Input: dimensioned drawing with shaded views. Units: mm. Origin: part minimum x, y, z. A direction names the side the tool comes from. Give positions to 0.01 mm unless a question says otherwise; leave off trailing zeros. Loops run counter-clockwise (first coordinate to the right, second up) from the corner with the lowest first, then second, coordinate; pieces in that order, holes last. Notation, with made-up numbers: M 31,34.5 L 88,34.5 A18 cw 88,44.5 Z; hole C -13.75,59 d9. An arc over 180 degrees is marked long. Answer in a Markdown table with one row per item.
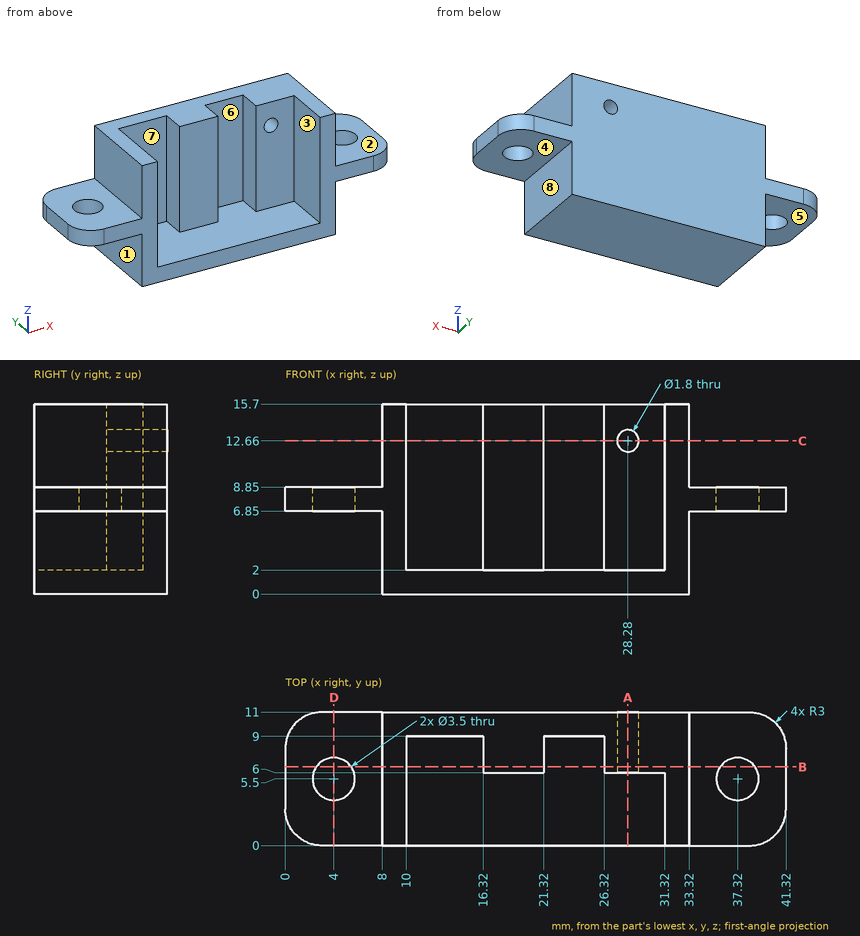
Q1. Section query B-B (y = 6.5). Give the number of separate pieces and of enclosed holes in the cut face, plus the area to 3 significant figures.
Values follow:
| item | result |
|---|---|
| separate pieces | 3 |
| enclosed holes | 1 |
| area | 260 mm^2 |
Q2. Ray query, probe 1 along X at (y, z) = (7.25, 9.25); probe 2 along Z at (x, y) = (28.28, 8.65); probe 3 along X at (y, z) = (3.5, 10.75). Return the intervals inside material, ascending. Write a range as from..to.
Values follow:
| item | result |
|---|---|
| probe 1 | 8..10, 16.32..21.32, 26.32..33.32 |
| probe 2 | 0..11.76, 13.56..15.7 |
| probe 3 | 8..10, 31.32..33.32 |
Q3. Contact query for flat-ended pins moving along their axis: pin 1 Ø4 at (x, z) = (28, 9.5) entering from -Y; pin 2 Ø5.5 at (y, z) = (6, 2.5) entering from -X; pin 3 Ø1.5 at (y, z) = (4, 12) entering from +X. Output: stop coordinate, or through.
Values follow:
| item | result |
|---|---|
| pin 1 | y = 6 |
| pin 2 | x = 8 |
| pin 3 | x = 33.32 |
Q4. Mould query, pull axis X, two halves, no side actions, for the marked faces 5, 6, 7 and 8. Classes: +X half, -X half, draft (parallel to the pull), parting line (faces both ways), or undercut.
Values follow:
| item | result |
|---|---|
| face 5 | draft |
| face 6 | undercut |
| face 7 | undercut |
| face 8 | +X half |
Q5. Section query C-C (z = 12.66). Output: boundary loops of the cut face in (x, y).
Values follow:
| item | result |
|---|---|
| outline | M 8,0 L 10,0 L 10,9 L 16.32,9 L 16.32,6 L 21.32,6 L 21.32,9 L 26.32,9 L 26.32,6 L 27.38,6 L 27.38,11 L 8,11 Z; M 29.18,6 L 31.32,6 L 31.32,0 L 33.32,0 L 33.32,11 L 29.18,11 Z |
Q6. Section query D-D (x = 4). Output: boundary loops of the cut face in (y, z).
Values follow:
| item | result |
|---|---|
| outline | M 0,6.85 L 3.75,6.85 L 3.75,8.85 L 0,8.85 Z; M 7.25,6.85 L 11,6.85 L 11,8.85 L 7.25,8.85 Z |
Q7. Reachability of the marked faces 1, 2, 3 and 4 from +Z, -Z, +X, -X, +Y, -Y: full face, straight path, thin tool, end or side. Return the list, or none.
Values follow:
| item | result |
|---|---|
| face 1 | -Z, -X, +Y, -Y |
| face 2 | +Z, +X, +Y, -Y |
| face 3 | +Z, -Y |
| face 4 | -Z, +X, +Y, -Y |
Q8. Section query A-A (x = 28.28). Output: boundary loops of the cut face in (y, z).
Values follow:
| item | result |
|---|---|
| outline | M 0,0 L 11,0 L 11,11.76 L 6,11.76 L 6,2 L 0,2 Z; M 6,13.56 L 11,13.56 L 11,15.7 L 6,15.7 Z |
